Here's how the part is built. I have some questions about the finished solid (model axes, mm). A direction names the side the tool comes from. Coordinates: 2 decimals unless noted, no trailing zeros. Loops run counter-clockwise (first coordinate to the right, second up) from the corner with the lowest first, then second, coordinate; pieces in that order, holes last. Notation, with made-up numbers: (40, 47.5) - (63, 47.5) arc R20 cw to (63, 54.5) - close; hole circle Ø2 at (-21, 42.5). An arc over 180 degrees is marked (long way). Use a Markdown table: item, result.
```python
from build123d import *

# Parameters (mm, degrees)
F1_DEPTH = 3.175
F2_DEPTH = 6.35
F0_W     = 13.1055872
F0_H     = 111.4425
F3_DEPTH = 11.684
F5_DEPTH = 113.03
F6_W     = 1.5875
F6_H     = 12.7
F7_DEPTH = 5.334


with BuildPart() as f1:
    # F0 (on Top) → F1 (new body)
    with BuildSketch(Plane.XY):
        Polygon((29.8689268, -55.72125), (29.8689268, 55.72125), (-29.8689268, 55.72125), (-29.8689268, -43.02125), (-15.1623268, -43.02125), (-15.1623268, -23.97125), (-8.8123268, -23.97125), (-8.8123268, -43.02125), (-8.8123268, -55.72125), align=None)
    extrude(amount=F1_DEPTH)

    # F0 (on Top) → F2 (join)
    with BuildSketch(Plane.XY):
        Polygon((-29.8689268, -43.02125), (-29.8689268, 55.72125), (-31.4564268, 55.72125), (-31.4564268, -55.72125), (-29.8689268, -55.72125), align=None)
    extrude(amount=F2_DEPTH)

    # F0 (on Top) → F3 (join)
    with BuildSketch(Plane.XY):
        Polygon((42.974514, -55.72125), (29.8689268, -55.72125), (-8.8123268, -55.72125), (-8.8123268, -57.30875), (42.974514, -57.30875), align=None)
        with Locations((36.4217204, 0)):
            Rectangle(F0_W, F0_H)
    extrude(amount=F3_DEPTH)

    # F4 (on face) → F5 (cut, through all)
    with BuildSketch(Plane(origin=(0, 55.72125, 0), x_dir=(-1, 0, 0), z_dir=(0, 1, 0))):
        Polygon((-42.974514, 0), (-29.8689268, 11.684), (-42.974514, 11.684), align=None)
    extrude(amount=-F5_DEPTH, mode=Mode.SUBTRACT)

    # F6 (on face) → F7 (join, through all)
    with BuildSketch(Plane.XY.offset(6.35)):
        with Locations((-30.6626768, 39.84625)):
            Rectangle(F6_W, F6_H)
        with Locations((-30.6626768, -43.02125)):
            Rectangle(F6_W, F6_H)
    extrude(amount=F7_DEPTH)


solid = f1.part
```
Q1. Which directions (+Z, -Z, +X, -X, +Y, -Y) give clear straight access to the entire face, cutting with the end or side of a thin tool? Please do faces 1 (the face through (0, 1, 3.175)), 2 (the face through (11, -57.309, 6)), 3 (the face through (-8.812, -42, 3)).
Check values:
| item | result |
|---|---|
| face 1 | +Z, +Y |
| face 2 | +Z, -Z, +X, -X, -Y |
| face 3 | +Z, -Z, -Y |
Q2. I want a section at D-D, the plane y = -5. Write out the boundary of the cut face in (x, z) (3 decimals).
Check values:
| item | result |
|---|---|
| outline | (-31.456, 0) - (42.975, 0) - (29.869, 11.684) - (29.869, 3.175) - (-29.869, 3.175) - (-29.869, 6.35) - (-31.456, 6.35) - close |
Q3. Will these pins go through, and if not, where does the flat tip stop? P1, Ø0.5, axis at x = -30.5, z = 10, coming from the -Y side; P2, Ø0.5, axis at x = -30.5, y = 49.5, coming from the +Z side; P3, Ø0.5, axis at x = -30.5, z = 10, coming from the +Y side.
Check values:
| item | result |
|---|---|
| P1 | y = -49.37 |
| P2 | z = 6.35 |
| P3 | y = 46.2 |
Q4. I want a section at C-C, the plane z = 4.5. Write out the boundary of the cut face in (x, y), then the cut area to 3 significant figures.
Check values:
| item | result |
|---|---|
| outline | (-31.46, -55.72) - (-29.87, -55.72) - (-29.87, 55.72) - (-31.46, 55.72) - close; (-8.81, -57.31) - (37.93, -57.31) - (37.93, 55.72) - (29.87, 55.72) - (29.87, -55.72) - (-8.81, -55.72) - close |
| area | 1,150 mm^2 |
Q5. I want a section at B-B, the plane z = 10.5. Write out the boundary of the cut face in (x, y), then the cut area to 3 significant figures.
Check values:
| item | result |
|---|---|
| outline | (-31.46, -49.37) - (-29.87, -49.37) - (-29.87, -36.67) - (-31.46, -36.67) - close; (-31.46, 33.5) - (-29.87, 33.5) - (-29.87, 46.2) - (-31.46, 46.2) - close; (-8.81, -57.31) - (31.2, -57.31) - (31.2, 55.72) - (29.87, 55.72) - (29.87, -55.72) - (-8.81, -55.72) - close |
| area | 252 mm^2 |
Q6. If we mould it in two halves opening along X, with no side actions, what happens to faces 4 (the face through (-31.456, 1, 4)), 5 (the face through (-12, -23.971, 2)), 6 (the face through (6, 55.721, 3))? For each: pulls with the +X half, pulls with the -X half, needs draft (parallel to the pull), parting line crosses it, or undercut.
Check values:
| item | result |
|---|---|
| face 4 | pulls with the -X half |
| face 5 | undercut |
| face 6 | needs draft |
Q7. I want a section at A-A, the plane y = -32. Write out the boundary of the cut face in (x, z) (3 decimals).
Check values:
| item | result |
|---|---|
| outline | (-31.456, 0) - (-15.162, 0) - (-15.162, 3.175) - (-29.869, 3.175) - (-29.869, 6.35) - (-31.456, 6.35) - close; (-8.812, 0) - (42.975, 0) - (29.869, 11.684) - (29.869, 3.175) - (-8.812, 3.175) - close |
Q8. Please list where these lines run through material, in increasing order: L1, parallel to Z at x = -18.5, y = 21 (3 decimals); L2, parallel to Y at x = 11, z = 10; L3, parallel to X at y = -48, z = 9. Write a range as from..to.
Check values:
| item | result |
|---|---|
| L1 | 0..3.175 |
| L2 | -57.31..-55.72 |
| L3 | -31.46..-29.87, 29.87..32.88 |
